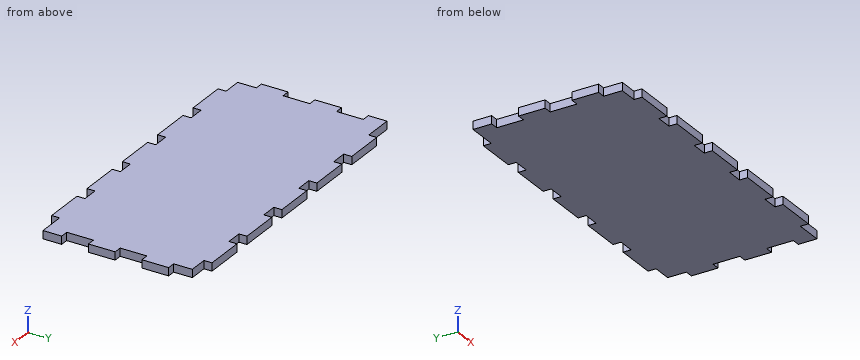
```python
from build123d import *

# Parameters (mm, degrees)
BOSS_EXTRUDE1_DEPTH = 3


with BuildPart() as part:
    # Sketch1 → Boss-Extrude1 (new body)
    with BuildSketch(Plane.XY):
        Polygon((120, 3), (120, 10), (117, 10), (117, 20), (120, 20), (120, 30), (117, 30), (117, 40), (120, 40), (120, 50), (117, 50), (117, 57), (110, 57), (110, 60), (95, 60), (95, 57), (89, 57), (89, 60), (74, 60), (74, 57), (68, 57), (68, 60), (53, 60), (53, 57), (47, 57), (47, 60), (32, 60), (32, 57), (26, 57), (26, 60), (11, 60), (11, 57), (5, 57), (0, 57), (0, 50), (3, 50), (3, 40), (0, 40), (0, 30), (3, 30), (3, 20), (0, 20), (0, 10), (3, 10), (3, 3), (10, 3), (10, 0), (25, 0), (25, 3), (31, 3), (31, 0), (46.25, 0), (46.25, 3), (52.25, 3), (52.25, 0), (67.5, 0), (67.5, 3), (73.5, 3), (73.5, 0), (88.75, 0), (88.75, 3), (94.75, 3), (94.75, 0), (110, 0), (110, 3), (116, 3), align=None)
    extrude(amount=BOSS_EXTRUDE1_DEPTH)


solid = part.part
```
Check sheet for the modelled part. Datum: model origin and axes. Units: mm. Round coordinates to 2 decimals unless told otherwise and drop trailing zeros. Loops run counter-clockwise (first coordinate to the right, second up) from the corner with the lowest first, then second, coordinate; pieces in that order, holes last. Notation, with made-up numbers: M 48,-32 L 63,-32 A20 cw 63,-18 Z; hole C -27.75,24.25 d1. An arc over 180 degrees is marked long. Answer as a JSON object with one key per item and string values.
1. Gauge pin test, flat ends, axial feed: P1, Ø1.5, axis at y = 26, z = 2, coming from the -X side; P2, Ø0.9, axis at y = 58.5, z = 1, coming from the -X side; P3, Ø1.5, axis at x = 108, z = 1.5, coming from the -Y side; P4, Ø1.5, axis at y = 59, z = 2, coming from the +X side. Record the tip position at first contact, or that the pin passes through.
Reply:
{"P1": "stops at x = 3", "P2": "stops at x = 11", "P3": "stops at y = 0", "P4": "stops at x = 110"}
2. Section check A-A (x = 92). Record the boundary of the cut face in (y, z).
Reply:
{"outline": "M 3,0 L 57,0 L 57,3 L 3,3 Z"}
3. Section check B-B (y = 46.5). Record the boundary of the cut face in (x, z).
Reply:
{"outline": "M 3,0 L 120,0 L 120,3 L 3,3 Z"}
4. Scan lines: line 1 (X direction, y = 18, z = 0.6); line 2 (X direction, y = 22.5, z = 1.35); line 3 (Y direction, x = 28.5, z = 1.75). Record each from-to range of solid material in increasing order.
Reply:
{"line 1": "x = 0 to 117", "line 2": "x = 3 to 120", "line 3": "y = 3 to 57"}
